Answer from the drawing. Dimensions are ordinates in mm from the lowest x, y and z of the part. Give positions to 0.01 mm unless a question says otherwise; leave off trailing zeros. Order: outer loops, then holes, each group sorted by start corner. A loop starts at its lowest first (then second) coordinate and runs counter-clockwise, first axis right, second up.
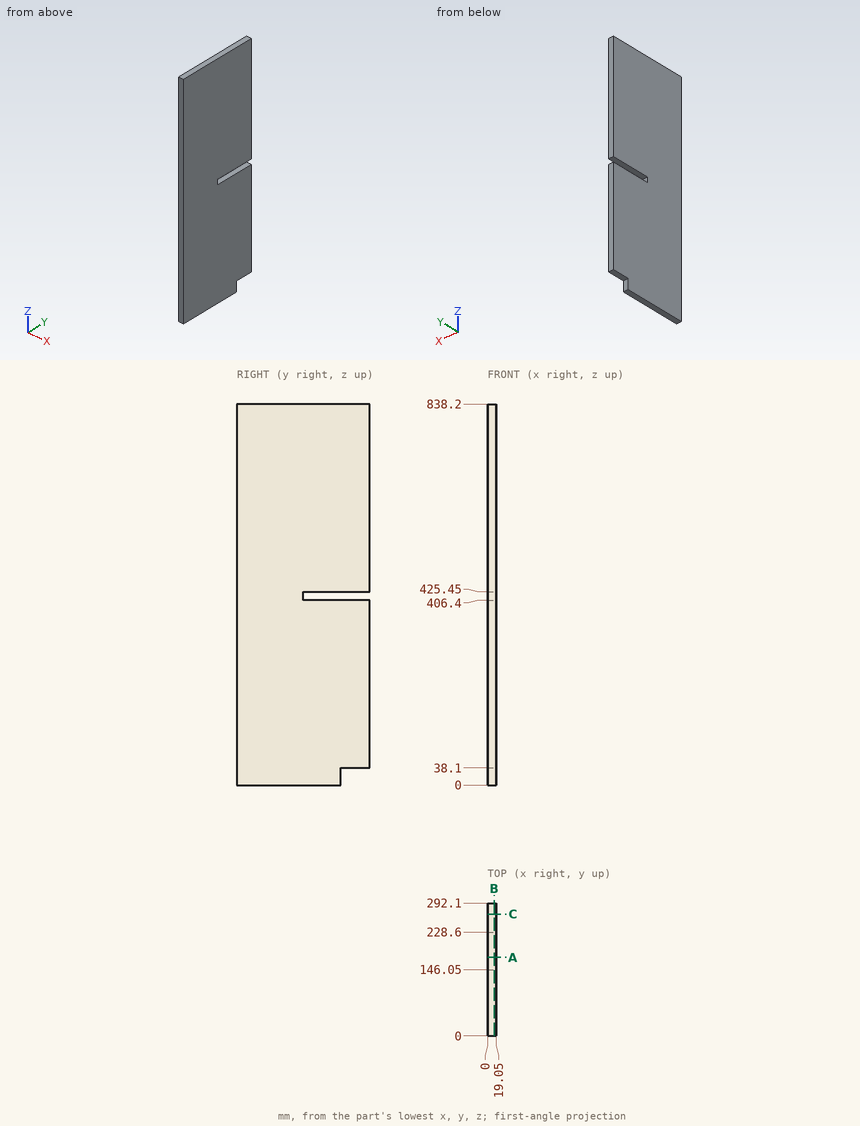
1) Given pin 1 (2 mm diameter, centred on y = 30.5, z = 579, fed in from -X); pin 2 (9.5 mm diameter, centred on x = 11.5, z = 12.5, fed in from +Y), each flat-ended and moving along its own axis, determine where each tip first touches the part or whether it passes through.
Final values:
pin 1: stops at x = 0
pin 2: stops at y = 228.6
2) The part is cut by section B-B on x = 14.25. Determine the outline of the cut face in (y, z), and give its area (3 significant figures).
Final values:
outline: (0, 0) - (228.6, 0) - (228.6, 38.1) - (292.1, 38.1) - (292.1, 406.4) - (146.05, 406.4) - (146.05, 425.45) - (292.1, 425.45) - (292.1, 838.2) - (0, 838.2) - close
area: 240,000 mm2
3) The part is cut by section A-A on y = 173. Determine the outline of the cut face in (x, z), and give its area (3 significant figures).
Final values:
outline: (0, 0) - (19.05, 0) - (19.05, 406.4) - (0, 406.4) - close; (0, 425.45) - (19.05, 425.45) - (19.05, 838.2) - (0, 838.2) - close
area: 15,600 mm2
4) Consider L1, parallel to Z at x = 6, y = 174; L2, parallel to Z at x = 14.5, y = 275; L3, parallel to Y at x = 11.5, z = 409. Determine where each line is inside the solid, lowest interval first.
Final values:
L1: z = 0 to 406.4, 425.45 to 838.2
L2: z = 38.1 to 406.4, 425.45 to 838.2
L3: y = 0 to 146.05
5) The part is cut by section C-C on y = 268. Determine the outline of the cut face in (x, z), and give its area (3 significant figures).
Final values:
outline: (0, 38.1) - (19.05, 38.1) - (19.05, 406.4) - (0, 406.4) - close; (0, 425.45) - (19.05, 425.45) - (19.05, 838.2) - (0, 838.2) - close
area: 14,900 mm2
